The model under review builds one solid part; all positions refer to its coordinate system, in mm. A direction names the side the tool comes from. Give positions to 0.01 mm unless a question says otherwise; leave off trailing zeros. Write each loop counter-clockwise with the first axis right and the second up, starting at its lowest first coordinate (ties: lowest second). Pieces come first, ordered by that corner, then holes.
from build123d import *

# Parameters (mm, degrees)
SKETCH1_W           = 45
SKETCH1_H           = 40
BOSS_EXTRUDE1_DEPTH = 6
SKETCH2_W           = 5
SKETCH2_H           = 5
SKETCH2_H_2         = 7
CUT_EXTRUDE1_DEPTH  = 6
SKETCH3_W           = 5
SKETCH3_H           = 5
SKETCH3_H_2         = 7
CUT_EXTRUDE3_DEPTH  = 6
SKETCH3_4_W         = 5
SKETCH3_4_H         = 5
SKETCH3_4_H_2       = 7
BOSS_EXTRUDE3_DEPTH = 6
SKETCH3_5_W         = 5
SKETCH3_5_H         = 10
SKETCH3_5_H_2       = 3
SKETCH3_5_H_3       = 5
CUT_EXTRUDE4_DEPTH  = 6
SKETCH4_W           = 5
SKETCH4_H           = 2
CUT_EXTRUDE10_DEPTH = 10
SKETCH5_W           = 5
SKETCH5_H           = 5
BOSS_EXTRUDE4_DEPTH = 6


with BuildPart() as part:
    # Sketch1 → Boss-Extrude1 (new body)
    with BuildSketch(Plane.XY):
        with Locations((4.06626506, -2.515060241)):
            Rectangle(SKETCH1_W, SKETCH1_H)
    extrude(amount=BOSS_EXTRUDE1_DEPTH)

    # Sketch2 → Cut-Extrude1 (cut)
    with BuildSketch(Plane.XY.offset(6)):
        with Locations((-15.93373494, 4.984939759)):
            Rectangle(SKETCH2_W, SKETCH2_H)
        with Locations((-15.93373494, -6.015060241)):
            Rectangle(SKETCH2_W, SKETCH2_H_2)
        with Locations((-15.93373494, -15.015060241)):
            Rectangle(SKETCH2_W, SKETCH2_H)
    extrude(amount=-CUT_EXTRUDE1_DEPTH, mode=Mode.SUBTRACT)

    # Sketch3 → Cut-Extrude3 (cut)
    with BuildSketch(Plane.XY.offset(6)):
        with Locations((24.06626506, -15.015060241)):
            Rectangle(SKETCH3_W, SKETCH3_H)
        with Locations((24.06626506, -4.015060241)):
            Rectangle(SKETCH3_W, SKETCH3_H_2)
        with Locations((24.06626506, 4.984939759)):
            Rectangle(SKETCH3_W, SKETCH3_H)
    extrude(amount=-CUT_EXTRUDE3_DEPTH, mode=Mode.SUBTRACT)

    # Sketch3<4> → Boss-Extrude3 (add)
    with BuildSketch(Plane.XY.offset(6)):
        with Locations((24.06626506, 4.984939759)):
            Rectangle(SKETCH3_4_W, SKETCH3_4_H)
        with Locations((24.06626506, -4.015060241)):
            Rectangle(SKETCH3_4_W, SKETCH3_4_H_2)
        with Locations((24.06626506, -15.015060241)):
            Rectangle(SKETCH3_4_W, SKETCH3_4_H)
    extrude(amount=-BOSS_EXTRUDE3_DEPTH)

    # Sketch3<5> → Cut-Extrude4 (cut)
    with BuildSketch(Plane.XY.offset(6)):
        with Locations((24.06626506, 12.484939759)):
            Rectangle(SKETCH3_5_W, SKETCH3_5_H)
        with Locations((24.06626506, 0.984939759)):
            Rectangle(SKETCH3_5_W, SKETCH3_5_H_2)
        with Locations((24.06626506, -10.015060241)):
            Rectangle(SKETCH3_5_W, SKETCH3_5_H_3)
        with Locations((24.06626506, -20.015060241)):
            Rectangle(SKETCH3_5_W, SKETCH3_5_H_3)
    extrude(amount=-CUT_EXTRUDE4_DEPTH, mode=Mode.SUBTRACT)

    # Sketch4 → Cut-Extrude10 (cut)
    with BuildSketch(Plane.XY.offset(6)):
        with Locations((-15.93373494, -1.515060241)):
            Rectangle(SKETCH4_W, SKETCH4_H)
    extrude(amount=-CUT_EXTRUDE10_DEPTH, mode=Mode.SUBTRACT)

    # Sketch5 → Boss-Extrude4 (add)
    with BuildSketch(Plane.XY.offset(6)):
        with Locations((-15.93373494, -10.015060241)):
            Rectangle(SKETCH5_W, SKETCH5_H)
    extrude(amount=-BOSS_EXTRUDE4_DEPTH)


solid = part.part
1) Insertion check: pin 1 (2.5 mm diameter, centred on x = 24.5, z = 4, fed in from +Y); pin 2 (1.5 mm diameter, centred on y = 5.5, z = 1.5, fed in from -X); pin 3 (2.5 mm diameter, centred on x = 23, z = 2.5, fed in from -Y). Each pin has a flat end and moves straight along its axis. Give the tip position at first contact, or say it passes through.
2) Tool access review of faces 1 (the flat face through (24, -12.515, 3)), 2 (the flat face through (26.566, -4, 3)), 3 (the flat face through (21.566, -20, 3)), 4 (the flat face through (21.566, 12, 3)), 5 (the flat face through (-16, -12.515, 3)): name each direction out of +Z, -Z, +X, -X, +Y, -Y from which nothing blocks a thin tool from reaching the whole face with its end or side.
3) Consider section B-B, the plane z = 3.75. Give the boundary of the cut face in (x, y), then the cut area to 3 significant figures.
4) The part is to be moulded in two halves that separate along Y. For faces 6 (the flat face through (-16, -0.515, 3)), 7 (the flat face through (26.566, -15, 3)), 8 (the flat face through (1, 17.485, 3)), say which applies: +Y half, -Y half, draft (parallel to the pull), parting line (faces both ways), or undercut.
5) Consider section A-A, the plane x = -16. Give the boundary of the cut face in (y, z), then the cut area to 3 significant figures.
6) Consider section C-C, the plane y = 15.5. Give the boundary of the cut face in (x, z), then the cut area to 3 significant figures.
7) To check wall thickness, follow probe 1 along Y at (x, z) = (22.5, 3.7); probe 2 along X at (y, z) = (8.5, 3.3); probe 3 along X at (y, z) = (-2.5, 0.65). State the ranges of each line that lie inside material, in increasing order.
Answer block:
1. pin 1: stops at y = 7.48
1. pin 2: stops at x = -13.43
1. pin 3: stops at y = -17.52
2. face 1: +Z, -Z, +X
2. face 2: +Z, -Z, +X, +Y, -Y
2. face 3: +Z, -Z, +X, -Y
2. face 4: +Z, -Z, +X, +Y
2. face 5: +Z, -Z, -X
3. outline: (-18.43, -22.52) - (21.57, -22.52) - (21.57, -17.52) - (26.57, -17.52) - (26.57, -12.52) - (21.57, -12.52) - (21.57, -7.52) - (26.57, -7.52) - (26.57, -0.52) - (21.57, -0.52) - (21.57, 2.48) - (26.57, 2.48) - (26.57, 7.48) - (21.57, 7.48) - (21.57, 17.48) - (-18.43, 17.48) - (-18.43, 7.48) - (-13.43, 7.48) - (-13.43, 2.48) - (-18.43, 2.48) - (-18.43, -0.52) - (-13.43, -0.52) - (-13.43, -7.52) - (-18.43, -7.52) - (-18.43, -12.52) - (-13.43, -12.52) - (-13.43, -17.52) - (-18.43, -17.52) - close
3. area: 1,600 mm2
4. face 6: undercut
4. face 7: draft
4. face 8: +Y half
5. outline: (-22.52, 0) - (-17.52, 0) - (-17.52, 6) - (-22.52, 6) - close; (-12.52, 0) - (-7.52, 0) - (-7.52, 6) - (-12.52, 6) - close; (-0.52, 0) - (2.48, 0) - (2.48, 6) - (-0.52, 6) - close; (7.48, 0) - (17.48, 0) - (17.48, 6) - (7.48, 6) - close
5. area: 138 mm2
6. outline: (-18.43, 0) - (21.57, 0) - (21.57, 6) - (-18.43, 6) - close
6. area: 240 mm2
7. probe 1: y = -17.52 to -12.52, -7.52 to -0.52, 2.48 to 7.48
7. probe 2: x = -18.43 to 21.57
7. probe 3: x = -13.43 to 26.57
